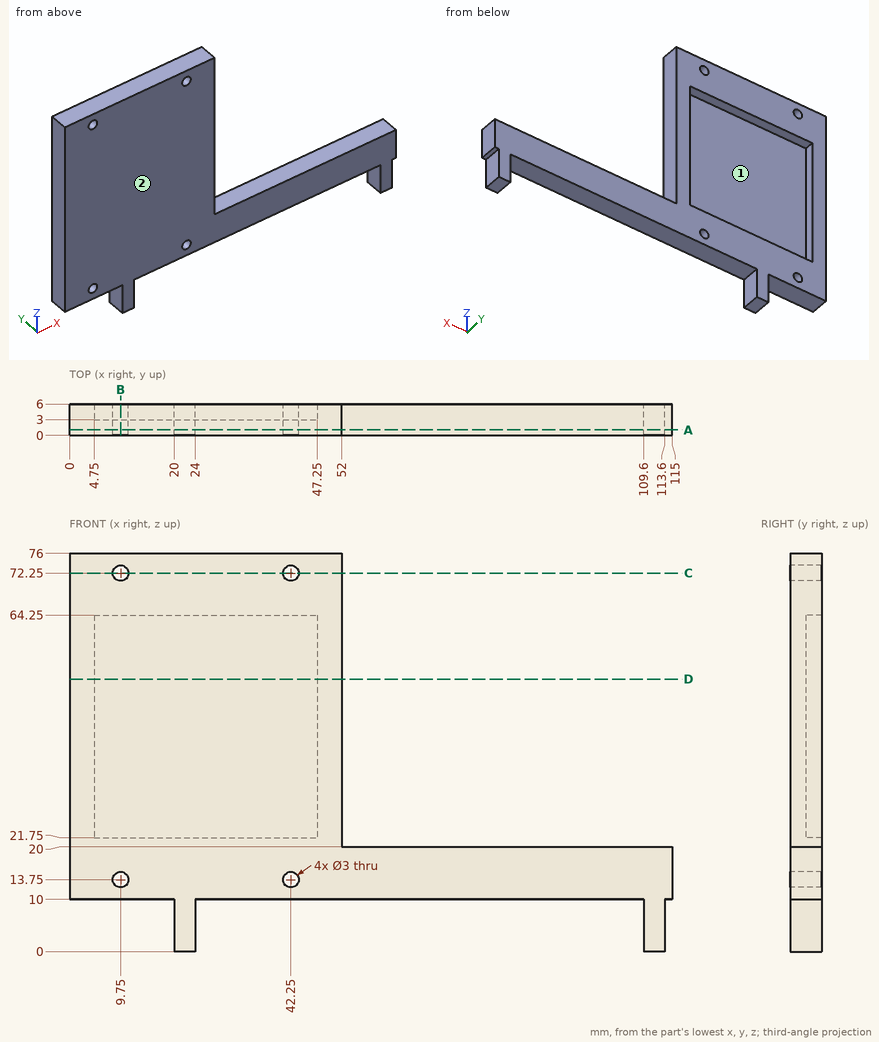
Geometry: see drawing. Coordinates: mm, zero at the bounding-box minimum. Coordinates: 2 decimals unless noted, no trailing zeros. Write each loop counter-clockwise with the first axis right and the second up, starting at its lowest first coordinate (ties: lowest second). Pieces come first, ordered by that corner, then holes.
1) Section D-D on z = 52. Output: boundary loops of the cut face in (x, y).
2) Material intervals for line 1 along X through (y, z) = (1.6, 72.25); line 2 along X through (y, z) = (3.5, 13.75); line 3 along Z through (x, y) = (27.5, 4.65), sorted ascending.
3) Section A-A on y = 1.05. Output: boundary loops of the cut face in (x, z).
4) Section C-C on z = 72.25. Output: boundary loops of the cut face in (x, y), and give its area (3 significant figures).
5) Mould query, pull axis X, two halves, no side actions, for the marked faces 1 and 2. Classes: pulls with the +X half, pulls with the -X half, needs draft (parallel to the pull), parting line crosses it, or undercut.
6) Pin query (flat end, axial travel): pin 1 Ø1.5 at (y, z) = (5, 42.5) entering from -X; pin 2 Ø1.8 at (y, z) = (3.5, 2.5) entering from +X; pin 3 Ø1.8 at (x, y) = (7, 3) entering from -Z; pin 4 Ø10 at (x, z) = (39, 57) entering from +Y. Return the tip coordinate at first contact, or that it passes through.
7) Section B-B on x = 9.75. Output: boundary loops of the cut face in (y, z).
Check result:
1. outline: (0, 0) - (52, 0) - (52, 6) - (47.25, 6) - (47.25, 3) - (4.75, 3) - (4.75, 6) - (0, 6) - close
2. line 1: x = 0 to 8.25, 11.25 to 40.75, 43.75 to 52
2. line 2: x = 0 to 8.25, 11.25 to 40.75, 43.75 to 115
2. line 3: z = 10 to 21.75, 64.25 to 76
3. outline: (0, 10) - (20, 10) - (20, 0) - (24, 0) - (24, 10) - (109.6, 10) - (109.6, 0) - (113.6, 0) - (113.6, 10) - (115, 10) - (115, 20) - (52, 20) - (52, 76) - (0, 76) - close; hole circle Ø3 at (9.75, 13.75); hole circle Ø3 at (9.75, 72.25); hole circle Ø3 at (42.25, 13.75); hole circle Ø3 at (42.25, 72.25)
4. outline: (0, 0) - (8.25, 0) - (8.25, 6) - (0, 6) - close; (11.25, 0) - (40.75, 0) - (40.75, 6) - (11.25, 6) - close; (43.75, 0) - (52, 0) - (52, 6) - (43.75, 6) - close
4. area: 276 mm2
5. face 1: undercut
5. face 2: needs draft
6. pin 1: stops at x = 0
6. pin 2: stops at x = 113.6
6. pin 3: stops at z = 10
6. pin 4: stops at y = 3
7. outline: (0, 10) - (6, 10) - (6, 12.25) - (0, 12.25) - close; (0, 15.25) - (6, 15.25) - (6, 21.75) - (3, 21.75) - (3, 64.25) - (6, 64.25) - (6, 70.75) - (0, 70.75) - close; (0, 73.75) - (6, 73.75) - (6, 76) - (0, 76) - close
